The figure shows three views and two pictorial views of one solid part (mm, origin at its lowest corner). Answer the questions. A direction names the side the tool comes from. Round coordinates to 2 decimals unless told otherwise and drop trailing zeros. Loops run counter-clockwise (first coordinate to the right, second up) from the corner with the lowest first, then second, coordinate; pieces in that order, holes last. Notation, with made-up numbers: (-13.5, 77.5) -> (40.5, 77.5) arc R14 ccw to (40.5, 100.5) -> close; hole circle Ø10 at (35, -14.75). An arc over 180 degrees is marked (long way). Use a Markdown table: item, result. Add a question column.
Q1. For a pull along Y with two mould halves and no side action, classify the marked faces 1, 2 and 3 as released by +Y, released by -Y, zero draft, split by the parting line, or undercut.
Q2. Section B-B on z = 4 is taken. Give the vertices of the cut face in (x, y).
Q3. Which of the six approach directions +Z, -Z, +X, -X, +Y, -Y give full straight-line access (tool end or side, diameter ignored) to the marked faces 4, 5 and 6?
Q4. Given pin 1 Ø1.5 at (y, z) = (35.5, 3) entering from -X; pin 2 Ø2.5 at (y, z) = (36, 5) entering from +X; pin 3 Ø1 at (x, z) = (19, 1) entering from +Y, each flat-ended and moving along its own axis, determine where each tip first touches the part or whether it passes through.
Q5. Section C-C on y = 10 is taken. Give the vertices of the cut face in (x, z).
Q6. Section D-D on x = 15 is taken. Give the vertices of the cut face in (y, z) (1 decimal), then the cut area to 3 significant figures.
Q7. Section A-A on x = 20 is taken. Give the vertices of the cut face in (y, z).
Q8. Consider line 1 (Z direction, x = 18, y = 10); line 2 (Y direction, x = 20, z = 2) (1 decimal); line 3 (Y direction, x = 19.5, z = 0.5) (1 decimal). Determine where each line is inside the solid, lowest interval first.
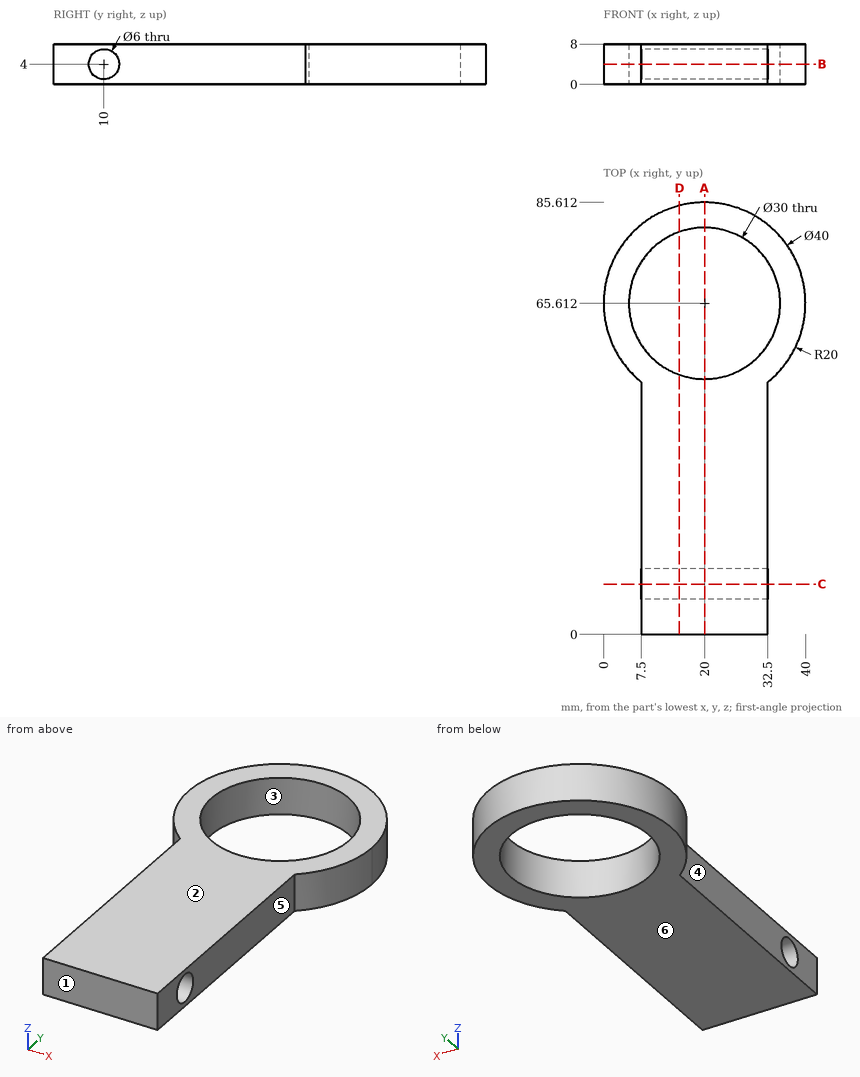
Checked values:
| question | item | result |
|---|---|---|
| 1 | face 1 | released by -Y |
| 1 | face 2 | zero draft |
| 1 | face 3 | undercut |
| 2 | outline | (7.5, 0) -> (32.5, 0) -> (32.5, 7) -> (7.5, 7) -> close; (7.5, 13) -> (32.5, 13) -> (32.5, 50) arc R20 ccw (long way) to (7.5, 50) -> close; hole circle Ø30 at (20, 65.61) |
| 3 | face 4 | +Z, -Z, -X, -Y |
| 3 | face 5 | +Z, -Z, +X, -Y |
| 3 | face 6 | -Z, +X, -X, +Y, -Y |
| 4 | pin 1 | stops at x = 7.5 |
| 4 | pin 2 | stops at x = 32.5 |
| 4 | pin 3 | stops at y = 85.61 |
| 5 | outline | (7.5, 0) -> (32.5, 0) -> (32.5, 1) -> (7.5, 1) -> close; (7.5, 7) -> (32.5, 7) -> (32.5, 8) -> (7.5, 8) -> close |
| 6 | outline | (0, 0) -> (51.5, 0) -> (51.5, 8) -> (0, 8) -> close; (79.8, 0) -> (85, 0) -> (85, 8) -> (79.8, 8) -> close; hole circle Ø6 at (10, 4) |
| 6 | area | 425 mm2 |
| 7 | outline | (0, 0) -> (50.61, 0) -> (50.61, 8) -> (0, 8) -> close; (80.61, 0) -> (85.61, 0) -> (85.61, 8) -> (80.61, 8) -> close; hole circle Ø6 at (10, 4) |
| 8 | line 1 | z = 0 to 1, 7 to 8 |
| 8 | line 2 | y = 0 to 7.8, 12.2 to 50.6, 80.6 to 85.6 |
| 8 | line 3 | y = 0 to 50.6, 80.6 to 85.6 |
